For this review, use the dimensioned drawing (mm, ordinates from the lowest corner) and the shaded views. Coordinates: 2 decimals unless noted, no trailing zeros. Loops run counter-clockwise (first coordinate to the right, second up) from the corner with the lowest first, then second, coordinate; pieces in that order, holes last. Notation, with made-up numbers: M 31,5 L 85,5 A19 cw 85,25 Z; hole C 47,24 d9. An arc over 180 degrees is marked long. Write item = value, one per line. Start each with the question number.
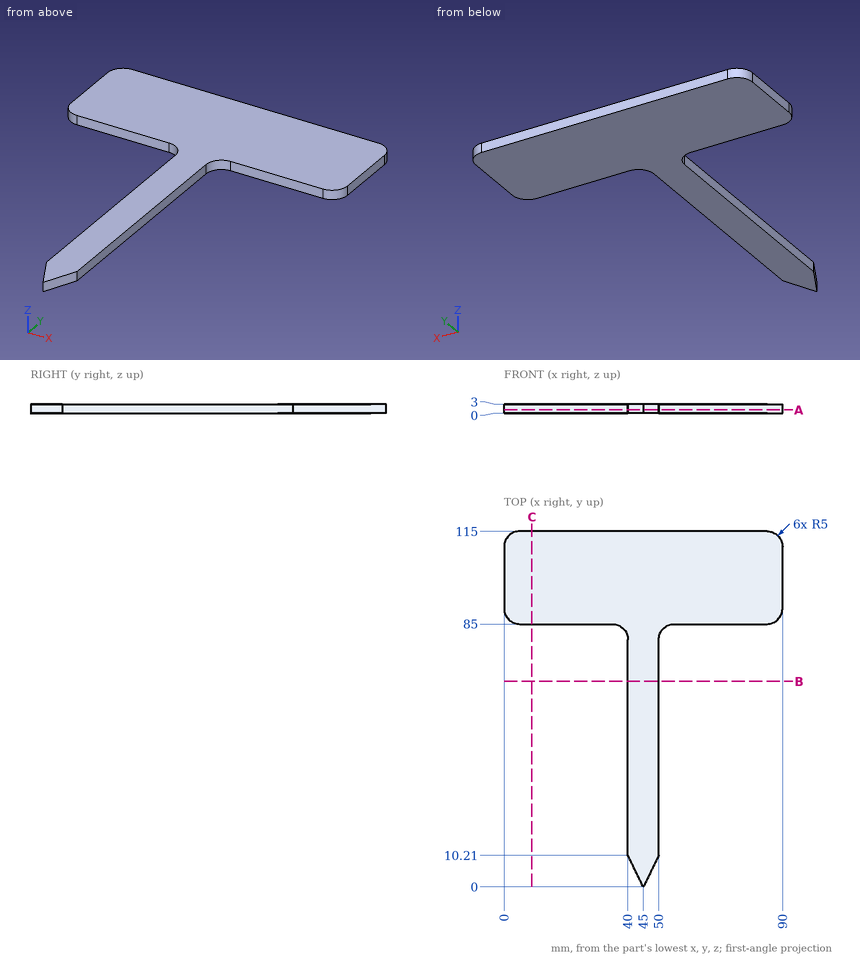
Q1. To check wall thickness, follow line 1 (Y direction, x = 56, z = 0.55); line 2 (X direction, y = 49, z = 2.55); line 3 (X direction, y = 6, z = 2.25). State the ranges of each line that lie inside material, in increasing order. Write a range as from..to.
Q2. Add section C-C on x = 9. State the section outline as (y, z) points.
Q3. Add section B-B on y = 66.5. State the section outline as (x, z) points.
Q4. Add section A-A on z = 1.1. State the section outline as (x, y) points, plus the area to 3 significant figures.
Q5. Clearance check with flat-ended pins moving along their axes: P1, Ø1, axis at y = 16, z = 2, coming from the +X side; P2, Ø0.9, axis at x = 14.5, z = 1.5, coming from the -Y side. State where each tip first meets the part, or that it passes through.
Values follow:
q1.line_1 = 85..115
q1.line_2 = 40..50
q1.line_3 = 42.06..47.94
q2.outline = M 85,0 L 115,0 L 115,3 L 85,3 Z
q3.outline = M 40,0 L 50,0 L 50,3 L 40,3 Z
q4.outline = M 0,90 A5 ccw 5,85 L 35,85 A5 cw 40,80 L 40,10.21 L 45,0 L 50,10.21 L 50,80 A5 cw 55,85 L 85,85 A5 ccw 90,90 L 90,110 A5 ccw 85,115 L 5,115 A5 ccw 0,110 Z
q4.area = 3,490 mm2
q5.P1 = 50
q5.P2 = 85
